Design review of the part built by this model. Coordinates are the model's own, in mm. Face numbers are marked on the shaded views. Round coordinates to 2 decimals unless told otherwise and drop trailing zeros. Loops run counter-clockwise (first coordinate to the right, second up) from the corner with the lowest first, then second, coordinate; pieces in that order, holes last. Notation, with made-up numbers: M 16,-15 L 72,-15 A20 ccw 72,2 Z; hole C 48,-38.75 d1. An arc over 180 degrees is marked long. Answer as CSV lines item,"result". Start each with the question number.
from build123d import *

# Parameters (mm, degrees)
F0_R         = 22.225
F1_DEPTH     = 19.05
F2_R         = 5.08
F3_T1_DEPTH  = 8.89
F3_S5_W      = 5.08
F3_S5_H      = 5.08
F3_T6_DEPTH  = 5.08
F3_S11_W     = 5.08
F3_S11_H     = 5.08
F3_T12_DEPTH = 5.08


# Not quite as in the source:
# - a fillet or chamfer that OpenCascade refuses, or shapes differently, is made with other operations: its cross-section is extruded or revolved along the edge and cut away or added


with BuildPart() as f1:
    # F0 (on Top) → F1 (new body)
    with BuildSketch(Plane.XY):
        Polygon((82.55, 0), (0, 0), (0, -19.05), (-57.8740507578, -19.05), (-76.2, -66.4293159973), (0, -66.4293159973), (0, -85.4793159973), (82.55, -85.4793159973), (82.55, -66.4293159973), (140.4240507578, -66.4293159973), (158.75, -19.05), (82.55, -19.05), align=None)
        with Locations((41.275, -42.7396579986)):
            Circle(F0_R, mode=Mode.SUBTRACT)
    extrude(amount=F1_DEPTH)

    # F2
    f2_edges = [f1.edges().sort_by_distance(p)[0] for p in [
        (111.487025, -66.429316, 19.05),
        (149.587025, -42.739658, 19.05),
        (120.65, -19.05, 19.05),
        (149.587025, -42.739658, 0),
        (111.487025, -66.429316, 0),
        (158.75, -19.05, 9.525),
        (140.424051, -66.429316, 9.525),
        (82.55, -75.954316, 19.05),
        (82.55, -85.479316, 9.525),
        (82.55, -75.954316, 0),
        (41.275, -85.479316, 0),
        (41.275, -85.479316, 19.05),
        (0, -75.954316, 19.05),
        (0, -75.954316, 0),
        (-38.1, -66.429316, 19.05),
        (-76.2, -66.429316, 9.525),
        (-38.1, -66.429316, 0),
        (-67.037025, -42.739658, 19.05),
        (-67.037025, -42.739658, 0),
        (-57.874051, -19.05, 9.525),
        (-28.937025, -19.05, 0),
        (-28.937025, -19.05, 19.05),
        (0, -9.525, 19.05),
        (0, 0, 9.525),
        (0, -9.525, 0),
        (41.275, 0, 19.05),
        (41.275, 0, 0),
        (82.55, -9.525, 19.05),
        (82.55, -9.525, 0),
        (120.65, -19.05, 0),
        (82.55, 0, 9.525),
    ]]
    fillet(f2_edges, radius=F2_R)

    # F3: fillet of radius 5.08 on 1 edges, made by hand

    # F3_s2 → F3_t1 (cut)
    with BuildSketch(Plane.XY.offset(5.08)):
        with BuildLine():
            ThreePointArc((5.08, -85.4793159973), (1.4878975516, -83.9914184457), (0, -80.3993159973))
            Line((0, -80.3993159973), (0, -85.4793159973))
            Line((0, -85.4793159973), (5.08, -85.4793159973))
        make_face()
    extrude(amount=F3_T1_DEPTH, mode=Mode.SUBTRACT)


with BuildPart() as f3_tool4:
    # F3_s5 → F3_t6 (new body)
    with BuildSketch(Plane.XZ.offset(80.3993159973)):
        with Locations((2.54, 2.54)):
            Rectangle(F3_S5_W, F3_S5_H)
    extrude(amount=F3_T6_DEPTH)

    # F3_s7 → F3_t8 (revolve, cut)
    with BuildSketch(Plane(origin=(5.08, -80.3993159973, 5.08), x_dir=(0.7071067812, 0, 0.7071067812), z_dir=(0.7071067812, 0, -0.7071067812))):
        with BuildLine():
            ThreePointArc((0, -5.08), (5.08, 0), (0, 5.08))
            Line((0, 5.08), (0, -5.08))
        make_face()
    revolve(axis=Axis((5.08, -80.3993159973, 5.08), (0, -1, 0)), mode=Mode.SUBTRACT)


with BuildPart() as f1_1:
    add(f1.part)

    # F3_t3: cut F3_tool4
    add(f3_tool4.part, mode=Mode.SUBTRACT)


with BuildPart() as f3_tool10:
    # F3_s11 → F3_t12 (new body)
    with BuildSketch(Plane.XZ.offset(80.3993159973)):
        with Locations((2.54, 16.51)):
            Rectangle(F3_S11_W, F3_S11_H)
    extrude(amount=F3_T12_DEPTH)

    # F3_s13 → F3_t14 (revolve, cut)
    with BuildSketch(Plane(origin=(5.08, -80.3993159973, 13.97), x_dir=(0.7071067812, 0, -0.7071067812), z_dir=(-0.7071067812, 0, -0.7071067812))):
        with BuildLine():
            ThreePointArc((0, -5.08), (5.08, 0), (0, 5.08))
            Line((0, 5.08), (0, -5.08))
        make_face()
    revolve(axis=Axis((5.08, -80.3993159973, 13.97), (0, -1, 0)), mode=Mode.SUBTRACT)


with BuildPart() as f1_2:
    add(f1_1.part)

    # F3_t9: cut F3_tool10
    add(f3_tool10.part, mode=Mode.SUBTRACT)


solid = f1_2.part
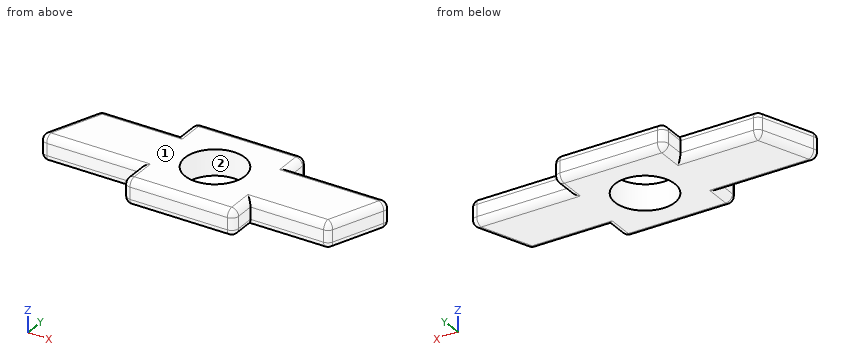
Item 1: Consider section C-C, the plane z = 16. Write out the cut boundary in (x, y) (3 decimals), then the cut area to 3 significant figures.
Item 2: To check wall thickness, follow line 1 (X direction, y = -17.5, z = 5.5); line 2 (Y direction, x = 89.5, z = 11.75); line 3 (Y direction, x = -2, z = 17.5). State the ranges of each line that lie inside material, in increasing order.
Item 3: The part is to be moulded in two halves that separate along Y. For the marked faces 1 and 2, say which applies: +Y half, -Y half, draft (parallel to the pull), parting line (faces both ways), or undercut.
Item 4: Consider section B-B, the plane x = 34. Write out the cut boundary in (y, z).
Item 5: Consider section A-A, the plane x = -49.5. Write out the cut boundary in (y, z), then the cut area to 3 significant figures.
Item 6: Consider section D-D, the plane y = -10.5. Write out the cut boundary in (x, z), then the cut area to 3 significant figures.
Item 7: Insertion check: pin 1 Ø6 at (y, z) = (-46, 7.5) entering from +X; pin 2 Ø2 at (x, z) = (90, 9) entering from +Y; pin 3 Ø7 at (y, z) = (-9.5, 8) entering from -X. Each pin has a flat end and moves straight along its axis. Give the tip position at first contact, or say it passes through.
Found:
1,outline,"M -73.132,-59.669 A4.657 ccw -68.788,-66.006 L 0.423,-66.006 L 0.423,-80.399 A4.657 ccw 5.08,-85.056 L 77.47,-85.056 A4.657 ccw 82.127,-80.399 L 82.127,-66.006 L 136.942,-66.006 A4.657 ccw 141.285,-63.029 L 155.682,-25.81 A4.657 ccw 151.338,-19.473 L 82.127,-19.473 L 82.127,-5.08 A4.657 ccw 77.47,-0.423 L 5.08,-0.423 A4.657 ccw 0.423,-5.08 L 0.423,-19.473 L -54.392,-19.473 A4.657 ccw -58.735,-22.45 Z; hole C 41.275,-42.74 d44.45"
1,area,"11,600 mm^2"
2,line 1,"x = 0 to 82.55"
2,line 2,"y = -66.43 to -19.05"
2,line 3,"y = -65 to -20.48"
3,face 1,"draft"
3,face 2,"undercut"
4,outline,"M -85.48,5.08 A5.08 ccw -80.4,0 L -63.74,0 L -63.74,19.05 L -80.4,19.05 A5.08 ccw -85.48,13.97 Z; M -21.74,0 L -5.08,0 A5.08 ccw 0,5.08 L 0,13.97 A5.08 ccw -5.08,19.05 L -21.74,19.05 Z"
5,outline,"M -66.43,5.08 A5.08 ccw -61.35,0 L -24.13,0 A5.08 ccw -19.05,5.08 L -19.05,13.97 A5.08 ccw -24.13,19.05 L -61.35,19.05 A5.08 ccw -66.43,13.97 Z"
5,area,"880 mm^2"
6,outline,"M 0,5.08 A5.08 ccw 5.08,0 L 77.47,0 A5.08 ccw 82.55,5.08 L 82.55,13.97 A5.08 ccw 77.47,19.05 L 5.08,19.05 A5.08 ccw 0,13.97 Z"
6,area,"1,550 mm^2"
7,pin 1,"stops at x = 149.49"
7,pin 2,"stops at y = -19.05"
7,pin 3,"stops at x = 0"
